from build123d import *

# Parameters (mm, degrees)
ESQUISSE1_R             = 4
BOSS_EXTRU_1_DEPTH      = 20
ESQUISSE2_W             = 10
ESQUISSE2_H             = 40
ENL_V_MAT_EXTRU_1_DEPTH = 20


with BuildPart() as part:
    # Esquisse1 → Boss.-Extru.1 (new body)
    with BuildSketch(Plane.XY):
        with BuildLine():
            Line((0, 20), (180, 20))
            ThreePointArc((180, 20), (200, 0), (180, -20))
            Line((180, -20), (0, -20))
            ThreePointArc((0, -20), (-20, 0), (0, 20))
        make_face()
        Circle(ESQUISSE1_R, mode=Mode.SUBTRACT)
        with Locations((180, 0)):
            Circle(ESQUISSE1_R, mode=Mode.SUBTRACT)
    extrude(amount=BOSS_EXTRU_1_DEPTH)

    # Esquisse2 → Enlèv. mat.-Extru.1 (cut, symmetric)
    with BuildSketch(Plane(origin=(0, 0, 0), x_dir=(0, 0, -1), z_dir=(1, 0, 0))):
        with Locations((-10, 0)):
            Rectangle(ESQUISSE2_W, ESQUISSE2_H)
    enl_v_mat_extru_1 = extrude(amount=ENL_V_MAT_EXTRU_1_DEPTH, both=True, mode=Mode.SUBTRACT)

    # Symétrie1: Enlèv. mat.-Extru.1 across plane
    add(enl_v_mat_extru_1.mirror(Plane(origin=(90, 0, 0), x_dir=(0, 0, 1), z_dir=(1, 0, 0))), mode=Mode.SUBTRACT)


solid = part.part
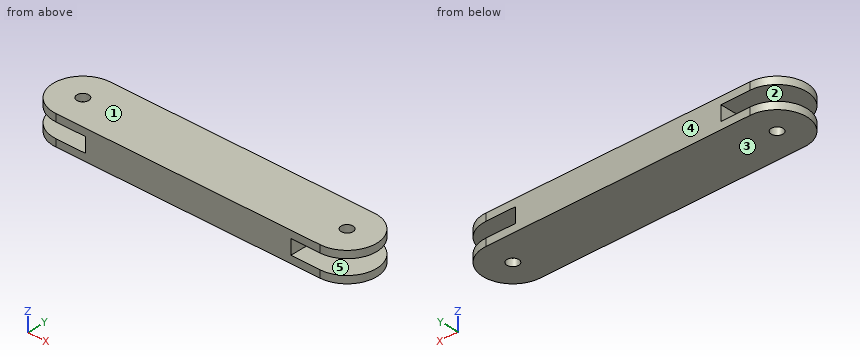
Verification items for the finished model (mm, model axes). Face numbers are marked on the shaded views. A direction names the side the tool comes from. Give positions to 0.01 mm unless a question says otherwise; leave off trailing zeros. Write each loop counter-clockwise with the first axis right and the second up, starting at its lowest first coordinate (ties: lowest second). Pieces come first, ordered by that corner, then holes. Notation, with made-up numbers: M 59,36.25 L 71,36.25 A30 cw 71,67.25 Z; hole C 58.5,52 d10. An arc over 180 degrees is marked long. Put each result on its own line as item: value. Start each with the question number.
1. Section check A-A (y = 0). Record the cut outline in (x, z), and give its area (3 significant figures).
2. Section check D-D (y = -11.5). Record the cut outline in (x, z).
3. Set-up check for the marked faces 4 and 5: record each of +Z, -Z, +X, -X, +Y, -Y from which the full face is reachable in a straight line by a thin tool's end or side.
4. Draft check along Z on the marked faces 1, 2 and 3. Enter one of: +Z half, -Z half, draft (parallel to the pull), parting line (faces both ways), or undercut.
5. Section check C-C (x = 186). Record the cut outline in (y, z).
6. Go/stop test with flat-tipped pins: pin 1 Ø12 at (x, y) = (182.5, -1.5) entering from -Z; pin 2 Ø6.5 at (x, y) = (0, 0) entering from -Z; pin 3 Ø11 at (y, z) = (-8.5, 9.5) entering from +X; pin 4 Ø10 at (y, z) = (-14.5, 17.5) entering from -X. Record where each tip stops, or that it passes through.
7. Section check B-B (y = 16). Record the cut outline in (x, z).
8. Scan lines: line 1 along X through (y, z) = (0, 17); line 2 along Z through (x, y) = (-3, 9); line 3 along Y through (x, z) = (0, 1.4). Record each from-to range of solid material in increasing order. Write a range as [from, to].
Answer list:
1. outline: M -20,0 L -4,0 L -4,5 L -20,5 Z; M -20,15 L -4,15 L -4,20 L -20,20 Z; M 4,0 L 176,0 L 176,5 L 160,5 L 160,15 L 176,15 L 176,20 L 4,20 L 4,15 L 20,15 L 20,5 L 4,5 Z; M 184,0 L 200,0 L 200,5 L 184,5 Z; M 184,15 L 200,15 L 200,20 L 184,20 Z
1. area: 3,440 mm2
2. outline: M -16.36,0 L 196.36,0 L 196.36,5 L 160,5 L 160,15 L 196.36,15 L 196.36,20 L -16.36,20 L -16.36,15 L 20,15 L 20,5 L -16.36,5 Z
3. face 4: +Z, -Z, +X, -X, +Y
3. face 5: +X, +Y, -Y
4. face 1: +Z half
4. face 2: undercut
4. face 3: -Z half
5. outline: M -19.08,0 L 19.08,0 L 19.08,5 L -19.08,5 Z; M -19.08,15 L 19.08,15 L 19.08,20 L -19.08,20 Z
6. pin 1: z = 0
6. pin 2: through
6. pin 3: x = 199.27
6. pin 4: x = -17.6
7. outline: M -12,0 L 192,0 L 192,5 L 160,5 L 160,15 L 192,15 L 192,20 L -12,20 L -12,15 L 20,15 L 20,5 L -12,5 Z
8. line 1: [-20, -4], [4, 176], [184, 200]
8. line 2: [0, 5], [15, 20]
8. line 3: [-20, -4], [4, 20]
